Model file for the job. Use its own axes, mm. Round coordinates to 2 decimals unless told otherwise and drop trailing zeros. Order: outer loops, then holes, each group sorted by start corner. A loop starts at its lowest first (then second) coordinate and runs counter-clockwise, first axis right, second up. Notation, with made-up numbers: (57, 0.5) - (70, 0.5) arc R20 ccw to (70, 23.5) - close; hole circle Ø11 at (87.25, -38.75). An arc over 180 degrees is marked (long way). Answer as CSV lines item,"result". Start each with the question number.
1. Pin check, flat tip, straight feed: pin 1 Ø1 at (x, z) = (-1.5, 1.5) entering from +Y. Stop position of the tip, or through.
2. Band-saw the part on B-B on y = 0.1. List the corners of the cut face in (x, z), then the cut area to 3 significant figures.
3. Band-saw the part on C-C on x = 1.65. List the corners of the cut face in (y, z).
4. Wall check: line 1 along Y through (x, z) = (1.15, 0.4); line 2 along X through (y, z) = (-0.05, 3.9); line 3 along X through (y, z) = (-0.7, 5.2). Give the ranges that are in metal, low to high. Write a range as [from, to].
5. Pull direction Y, two halves, no side cores. Call faces 1 (the face through (2, 0, 6)), 2 (the face through (-1.5, -0.07, 2.96)): released by +Y, released by -Y, zero draft, split by the parting line, or undercut.
6. Band-saw the part on A-A on y = 1.2. List the corners of the cut face in (x, z).
Autodesk Inventor part; units mm, degrees
ref_plane "YZ Plane" through (0, 0, 0) normal (1, 0, 0) x (0, 1, 0)
ref_plane "XZ Plane" through (0, 0, 0) normal (0, 1, 0) x (-1, 0, 0)
ref_plane "XY Plane" through (0, 0, 0) normal (0, 0, 1) x (1, 0, 0)
sketch "Sketch1" plane through (0, 0, 0) normal (0, 0, 1) x (1, 0, 0)
  circle A0 centre (0, 0) radius 1.5
  circle A1 centre (0, 0) radius 2.5 construction
  circle A2 centre (0, 0) radius 1.9
  line L0 (-0.7576, 1.7424) -> (0, 2.5)
  line L1 (0, 2.5) -> (0.7576, 1.7424)
  line L2 (0, 2.5) -> (0, 0) construction
  line L3 (-1.2589, 1.4231) -> (-0.7725, 2.3776)
  line L4 (-0.7725, 2.3776) -> (0.182, 1.8913)
  line L5 (-1.6371, 0.9644) -> (-1.4695, 2.0225)
  line L6 (-1.4695, 2.0225) -> (-0.4113, 1.8549)
  line L7 (-1.8549, 0.4113) -> (-2.0225, 1.4695)
  line L8 (-2.0225, 1.4695) -> (-0.9644, 1.6371)
  line L9 (-1.8913, -0.182) -> (-2.3776, 0.7725)
  line L10 (-2.3776, 0.7725) -> (-1.4231, 1.2589)
  line L11 (-1.7424, -0.7576) -> (-2.5, 0)
  line L12 (-2.5, 0) -> (-1.7424, 0.7576)
  line L13 (-1.4231, -1.2589) -> (-2.3776, -0.7725)
  line L14 (-2.3776, -0.7725) -> (-1.8913, 0.182)
  line L15 (-0.9644, -1.6371) -> (-2.0225, -1.4695)
  line L16 (-2.0225, -1.4695) -> (-1.8549, -0.4113)
  line L17 (-0.4113, -1.8549) -> (-1.4695, -2.0225)
  line L18 (-1.4695, -2.0225) -> (-1.6371, -0.9644)
  line L19 (0.182, -1.8913) -> (-0.7725, -2.3776)
  line L20 (-0.7725, -2.3776) -> (-1.2589, -1.4231)
  line L21 (0.7576, -1.7424) -> (0, -2.5)
  line L22 (0, -2.5) -> (-0.7576, -1.7424)
  line L23 (1.2589, -1.4231) -> (0.7725, -2.3776)
  line L24 (0.7725, -2.3776) -> (-0.182, -1.8913)
  line L25 (1.6371, -0.9644) -> (1.4695, -2.0225)
  line L26 (1.4695, -2.0225) -> (0.4113, -1.8549)
  line L27 (1.8549, -0.4113) -> (2.0225, -1.4695)
  line L28 (2.0225, -1.4695) -> (0.9644, -1.6371)
  line L29 (1.8913, 0.182) -> (2.3776, -0.7725)
  line L30 (2.3776, -0.7725) -> (1.4231, -1.2589)
  line L31 (1.7424, 0.7576) -> (2.5, 0)
  line L32 (2.5, 0) -> (1.7424, -0.7576)
  line L33 (1.4231, 1.2589) -> (2.3776, 0.7725)
  line L34 (2.3776, 0.7725) -> (1.8913, -0.182)
  line L35 (0.9644, 1.6371) -> (2.0225, 1.4695)
  line L36 (2.0225, 1.4695) -> (1.8549, 0.4113)
  line L37 (0.4113, 1.8549) -> (1.4695, 2.0225)
  line L38 (1.4695, 2.0225) -> (1.6371, 0.9644)
  line L39 (-0.182, 1.8913) -> (0.7725, 2.3776)
  line L40 (0.7725, 2.3776) -> (1.2589, 1.4231)
  point P0 (-0.992, 1.9469)
  point P1 (-1.5451, 1.5451)
  point P2 (-1.9469, 0.992)
  point P3 (-2.1582, 0.3418)
  point P4 (-2.1582, -0.3418)
  point P5 (-1.9469, -0.992)
  point P6 (-1.5451, -1.5451)
  point P7 (-0.992, -1.9469)
  point P8 (-0.3418, -2.1582)
  point P9 (0.3418, -2.1582)
  point P10 (0.992, -1.9469)
  point P11 (1.5451, -1.5451)
  point P12 (1.9469, -0.992)
  point P13 (2.1582, -0.3418)
  point P14 (2.1582, 0.3418)
  point P15 (1.9469, 0.992)
  point P16 (1.5451, 1.5451)
  point P17 (0.992, 1.9469)
  point P18 (0.3418, 2.1582)
  point P19 (-0.3418, 2.1582)
  dimension "d1" = 5
  dimension "d0" = 3
  dimension "d2" = 0.4
  dimension "d5" = 360
extrude "Extrusion1" add sketch "Sketch1" along normal blind 6
properties part number "fancy spacer"
Reply:
1,pin 1,"stops at y = 2.02"
2,outline,"(-2.4, 0) - (-1.5, 0) - (-1.5, 6) - (-2.4, 6) - close; (1.5, 0) - (2.4, 0) - (2.4, 6) - (1.5, 6) - close"
2,area,"10.8 mm2"
3,outline,"(-1.53, 0) - (1.53, 0) - (1.53, 6) - (-1.53, 6) - close"
4,line 1,"y = [-1.97, -0.96], [0.96, 1.97]"
4,line 2,"x = [-2.45, -1.5], [1.5, 2.45]"
4,line 3,"x = [-2.34, -1.33], [1.33, 2.34]"
5,face 1,"zero draft"
5,face 2,"undercut"
6,outline,"(-1.98, 0) - (-0.9, 0) - (-0.9, 6) - (-1.98, 6) - close; (0.9, 0) - (1.98, 0) - (1.98, 6) - (0.9, 6) - close"
